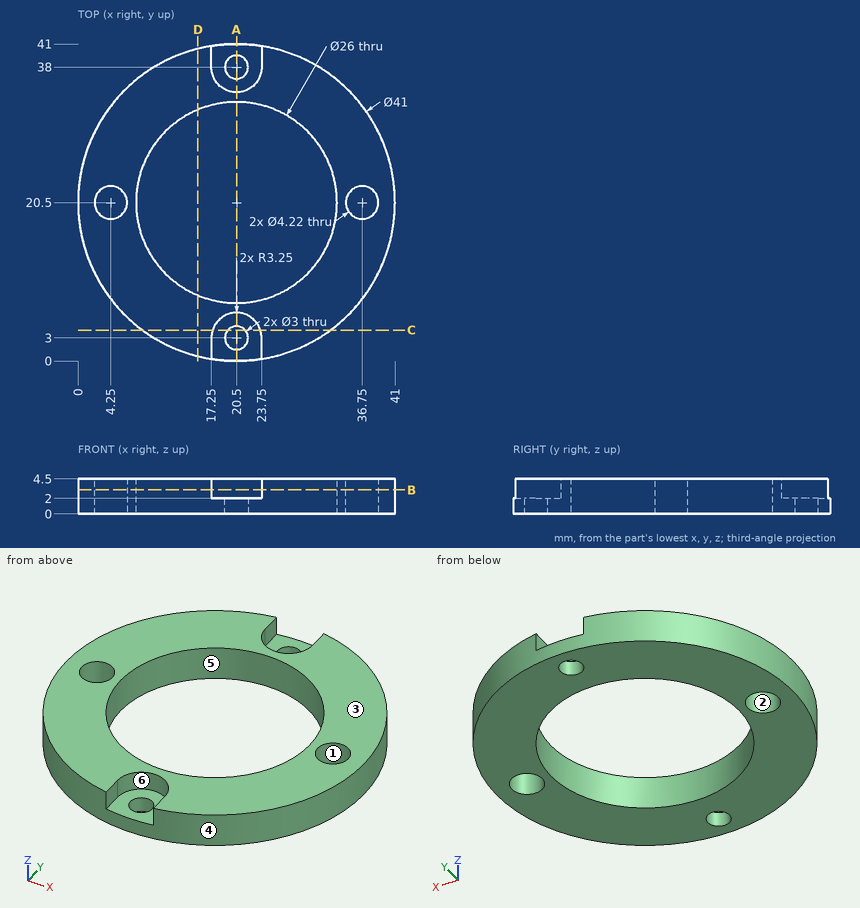
Verification items for this drawing (mm, ordinates from the low corner). A direction names the side the tool comes from. Round coordinates to 2 decimals unless told otherwise and drop trailing zeros. Write each loop counter-clockwise with the first axis right and the second up, starting at its lowest first coordinate (ties: lowest second). Pieces come first, ordered by that corner, then holes. Notation, with made-up numbers: M 21,75 L 78,75 A12 ccw 78,83 Z; hole C -16,-35 d5. An arc over 180 degrees is marked long. Write item = value, one per line. Start each with the question number.
1. Section check C-C, the plane y = 4. Record the cut outline in (x, z), then the cut area to 3 significant figures.
2. Tool access check on the marked faces 5 and 6. Record the directions out of +Z, -Z, +X, -X, +Y, -Y that give a thin tool (end or side, any length) a straight path to the whole face; none if there is none.
3. Scan lines: line 1 (Y direction, x = 20.5, z = 0.8); line 2 (Y direction, x = 12, z = 3); line 3 (X direction, y = 35, z = 3.6). Record each from-to range of solid material in increasing order. Write a range as [from, to].
4. Section check B-B, the plane z = 3.1. Record the cut outline in (x, y), then the cut area to 3 significant figures.
5. Section check A-A, the plane x = 20.5. Record the cut outline in (y, z).
6. Release check for a two-part mould opening along Y. For the marked faces 1, 2, 3 and 4 record: pulls with the +Y half, pulls with the -Y half, needs draft (parallel to the pull), parting line crosses it, or undercut.
7. Section check D-D, the plane x = 15.5. Record the cut outline in (y, z).
8. Gauge pin test, flat ends, axial feed: pin 1 (1.5 mm diameter, centred on x = 36.5, y = 5.5, fed in from +Z); pin 2 (1.2 mm diameter, centred on y = 39.5, z = 3, fed in from -X); pin 3 (1.9 mm diameter, centred on x = 20.5, y = 39, fed in from +Z); pin 4 (2 mm diameter, centred on y = 1.5, z = 3, fed in from +X). Record the tip position at first contact, or that the pin passes through.
Results found:
q1.outline = M 8.33,0 L 19.38,0 L 19.38,2 L 17.41,2 L 17.41,4.5 L 8.33,4.5 Z; M 21.62,0 L 32.67,0 L 32.67,4.5 L 23.59,4.5 L 23.59,2 L 21.62,2 Z
q1.area = 89.6 mm^2
q2.face_5 = +Z, -Z
q2.face_6 = +Z, -Y
q3.line_1 = [0, 1.5], [4.5, 7.5], [33.5, 36.5], [39.5, 41]
q3.line_2 = [1.85, 10.66], [30.34, 39.15]
q3.line_3 = [6.01, 19.25], [21.75, 34.99]
q4.outline = M 17.25,0.26 L 17.25,3 A3.25 cw 23.75,3 L 23.75,0.26 A20.5 ccw 23.75,40.74 L 23.75,38 A3.25 cw 17.25,38 L 17.25,40.74 A20.5 ccw Z; hole C 4.25,20.5 d4.22; hole C 20.5,20.5 d26; hole C 36.75,20.5 d4.22
q4.area = 690 mm^2
q5.outline = M 0,0 L 1.5,0 L 1.5,2 L 0,2 Z; M 4.5,0 L 7.5,0 L 7.5,4.5 L 6.25,4.5 L 6.25,2 L 4.5,2 Z; M 33.5,0 L 36.5,0 L 36.5,2 L 34.75,2 L 34.75,4.5 L 33.5,4.5 Z; M 39.5,0 L 41,0 L 41,2 L 39.5,2 Z
q6.face_1 = undercut
q6.face_2 = undercut
q6.face_3 = needs draft
q6.face_4 = parting line crosses it
q7.outline = M 0.62,0 L 8.5,0 L 8.5,4.5 L 0.62,4.5 Z; M 32.5,0 L 40.38,0 L 40.38,4.5 L 32.5,4.5 Z
q8.pin_1 = through
q8.pin_2 = 11.46
q8.pin_3 = 2
q8.pin_4 = 30.31
